Verification items for the finished model (mm, model axes). Face numbers are marked on the shaded views. Coordinates: 2 decimals unless noted, no trailing zeros. Write each loop counter-clockwise with the first axis right and the second up, starting at its lowest first coordinate (ties: lowest second). Pieces come first, ordered by that corner, then holes.
```python
from build123d import *

# Parameters (mm, degrees)
SKETCH_1_R          = 30
EXTRUDE_1_DEPTH     = 25.6
SKETCH_2_R          = 6
SKETCH_2_R_2        = 1.5
CUT_EXTRUDE_1_DEPTH = 30


with BuildPart() as part:
    # ｽｹｯﾁ1 → ﾎﾞｽ - 押し出し1 (new body)
    with BuildSketch(Plane(origin=(0, 0, 0), x_dir=(0, 0, -1), z_dir=(1, 0, 0))):
        Circle(SKETCH_1_R)
    extrude(amount=EXTRUDE_1_DEPTH)

    # ｽｹｯﾁ2 → ｶｯﾄ - 押し出し1 (cut)
    with BuildSketch(Plane.ZY):
        Circle(SKETCH_2_R)
        with Locations((10.5, 0)):
            Circle(SKETCH_2_R_2)
        with Locations((5.25, -9.09326674)):
            Circle(SKETCH_2_R_2)
        with Locations((-5.25, -9.09326674)):
            Circle(SKETCH_2_R_2)
        with Locations((-10.5, 0)):
            Circle(SKETCH_2_R_2)
        with Locations((-5.25, 9.09326674)):
            Circle(SKETCH_2_R_2)
        with Locations((5.25, 9.09326674)):
            Circle(SKETCH_2_R_2)
    extrude(amount=-CUT_EXTRUDE_1_DEPTH, mode=Mode.SUBTRACT)


solid = part.part
```
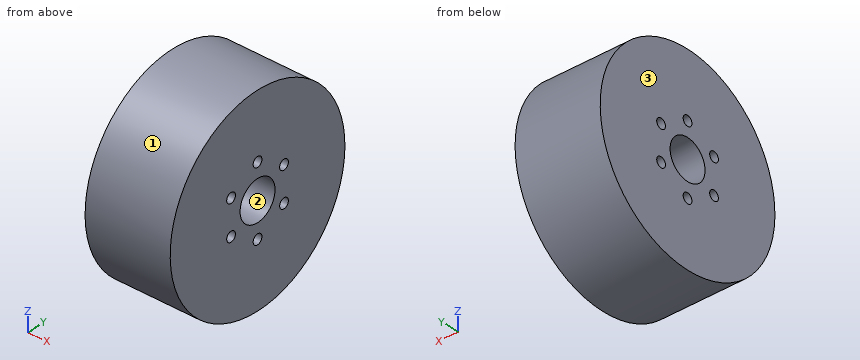
1. Material ranges on L1, parallel to Y at x = 19.25, z = 5.25; L2, parallel to Y at x = 8.25, z = 0; L3, parallel to Z at x = 9.25, y = -1, recorded low to high.
2. Sectioned sample at A-A, the plane z = 0. Record the boundary of the cut face in (x, y), and give its area (3 significant figures).
3. Sectioned sample at B-B, the plane y = 0. Record the boundary of the cut face in (x, z), and give its area (3 significant figures).
4. Sectioned sample at D-D, the plane z = -10.5. Record the boundary of the cut face in (x, y).
5. Sectioned sample at C-C, the plane x = 5.25. Record the boundary of the cut face in (y, z), and give its area (3 significant figures).
6. Draft check along Z on the marked faces 1, 2 and 3. Enter one of: pulls with the +Z half, pulls with the -Z half, needs draft (parallel to the pull), parting line crosses it, or undercut.
7. Gauge pin test, flat ends, axial feed: P1, Ø1, axis at x = 8.5, y = 12, coming from the +Z side; P2, Ø3, axis at x = 16.5, z = -1, coming from the +Y side; P3, Ø4, axis at x = 15.5, y = 2.5, coming from the +Z side. Record the tip position at first contact, or that the pin passes through.
Outcome:
1. L1: y = -29.54 to -10.59, -7.59 to -2.9, 2.9 to 7.59, 10.59 to 29.54
1. L2: y = -30 to -6, 6 to 30
1. L3: z = -29.98 to -11.62, -9.38 to -5.92, 5.92 to 9.38, 11.62 to 29.98
2. outline: (0, -30) - (25.6, -30) - (25.6, -6) - (0, -6) - close; (0, 6) - (25.6, 6) - (25.6, 30) - (0, 30) - close
2. area: 1,230 mm2
3. outline: (0, -30) - (25.6, -30) - (25.6, -12) - (0, -12) - close; (0, -9) - (25.6, -9) - (25.6, -6) - (0, -6) - close; (0, 6) - (25.6, 6) - (25.6, 9) - (0, 9) - close; (0, 12) - (25.6, 12) - (25.6, 30) - (0, 30) - close
3. area: 1,080 mm2
4. outline: (0, -28.1) - (25.6, -28.1) - (25.6, -1.5) - (0, -1.5) - close; (0, 1.5) - (25.6, 1.5) - (25.6, 28.1) - (0, 28.1) - close
5. outline: circle Ø60 at (0, 0); hole circle Ø3 at (-9.09, -5.25); hole circle Ø3 at (-9.09, 5.25); hole circle Ø12 at (0, 0); hole circle Ø3 at (0, -10.5); hole circle Ø3 at (0, 10.5); hole circle Ø3 at (9.09, -5.25); hole circle Ø3 at (9.09, 5.25)
5. area: 2,670 mm2
6. face 1: parting line crosses it
6. face 2: undercut
6. face 3: needs draft
7. P1: stops at z = 27.71
7. P2: stops at y = 30
7. P3: stops at z = 30
